Read the model definition and answer for the solid it produces. Units are mm, in the model's axes. A direction names the side the tool comes from. Round coordinates to 2 decimals unless told otherwise and drop trailing zeros. Write each loop counter-clockwise with the first axis right and the second up, starting at its lowest first coordinate (ties: lowest second). Pieces come first, ordered by that corner, then holes. Notation, with made-up numbers: (53.5, -14) - (99.5, -14) arc R7 ccw to (99.5, -2) - close; hole circle Ø4 at (80, 30). An arc over 180 degrees is marked (long way). One line per item, written item: value. Start each with the question number.
(1) The mould has two halves that part along X. Classify faces 6 (the face through (23.743, 55.535, -19.6)), 7 (the face through (-19, 53, 17)), 8 (the face through (-22.12, 55.26, -15.05)): +X half, -X half, draft (parallel to the pull), parting line (faces both ways), or undercut.
(2) A cutting plane is placed at B-B, the plane z = 0. Determine the outline of the cut face in (x, y).
(3) Find the intervals of material crossed by L1, parallel to X at y = 6.5, z = 0; L2, parallel to Y at x = -6.5, z = 21; L3, parallel to X at y = 4.25, z = -25, in increasing order.
(4) A cutting plane is placed at C-C, the plane x = -26. Determine the outline of the cut face in (y, z).
(5) For faces 1 (the face through (15.05, 55.26, -22.12)), 2 (the face through (0.66, 27.094, -14.985)), 3 (the face through (-5.865, 54.181, 14.366)), 4 (the face through (-18.684, 55.535, -19.6)), 5 (the face through (18.5, 53, 18.5)), determine the directions among +Z, -Z, +X, -X, +Y, -Y from which every point of the face is accessible in a straight line to the end or side of a thin tool.
(6) A cutting plane is placed at A-A, the plane x = 0. Determine the outline of the cut face in (y, z).
(7) A cutting plane is placed at D-D, the plane y = 51.5. Determine the outline of the cut face in (x, z).
(8) Flat-ended cylindrical pins translate along their axes: pin 1 Ø5.5 at (x, z) = (25, 0) entering from -Y; pin 2 Ø9.5 at (x, z) = (21.21, 21.21) entering from -Y; pin 3 Ø1.5 at (x, z) = (17.5, -5) entering from +Y; pin 4 Ø1 at (y, z) = (49.5, -5.5) entering from +X. Find the tip coordinate at first contact, or state that the pin passes through.
from build123d import *

# Parameters (mm, degrees)
SKETCH1_R           = 37.5
BOSS_EXTRUDE1_DEPTH = 8
SKETCH2_R           = 3
CUT_EXTRUDE1_DEPTH  = 54.633012222
SKETCH3_R           = 15
BOSS_EXTRUDE2_DEPTH = 50
BOSS_EXTRUDE4_START = -5
BOSS_EXTRUDE4_DEPTH = 5
CUT_EXTRUDE2_REACH  = 80.591
SKETCH5_R           = 3
FILLET1_R           = 5


with BuildPart() as part:
    # Sketch1 → Boss-Extrude1 (new body)
    with BuildSketch(Plane(origin=(0, 0, 0), x_dir=(1, 0, 0), z_dir=(0, 1, 0))):
        with Locations(Location((0, 0, 0), (0, 0, 270))):
            Circle(SKETCH1_R)
    extrude(amount=BOSS_EXTRUDE1_DEPTH)

    # Sketch2 → Cut-Extrude1 (cut, through all)
    with BuildSketch(Plane(origin=(0, 8, 0), x_dir=(1, 0, 0), z_dir=(0, 1, 0))):
        with Locations(Location((25, 0, 0), (0, 0, 270))):
            Circle(SKETCH2_R)
        with Locations(Location((0, 25, 0), (0, 0, 270))):
            Circle(SKETCH2_R)
        with Locations(Location((-25, 0, 0), (0, 0, 270))):
            Circle(SKETCH2_R)
        with Locations(Location((0, -25, 0), (0, 0, 270))):
            Circle(SKETCH2_R)
    extrude(amount=-CUT_EXTRUDE1_DEPTH, mode=Mode.SUBTRACT)

    # Sketch3 → Boss-Extrude2 (add)
    with BuildSketch(Plane(origin=(0, 8, 0), x_dir=(1, 0, 0), z_dir=(0, 1, 0))):
        with Locations(Location((0, 0, 0), (0, 0, 270))):
            Circle(SKETCH3_R)
    extrude(amount=BOSS_EXTRUDE2_DEPTH)

    # Sketch7 → Boss-Extrude4 (add)
    with BuildSketch(Plane(origin=(0, 58, 0), x_dir=(1, 0, 0), z_dir=(0, 1, 0)).offset(BOSS_EXTRUDE4_START)):
        with BuildLine():
            ThreePointArc((-6.464466094, -13.535533906), (-10.606601718, -10.606601718), (-13.535533906, -6.464466094))
            Line((-13.535533906, -6.464466094), (-28.284271247, -21.213203436))
            Line((-28.284271247, -21.213203436), (-21.213203436, -28.284271247))
            Line((-21.213203436, -28.284271247), (-6.464466094, -13.535533906))
        make_face()
        with BuildLine():
            Line((0, -7.071067812), (-7.071067812, 0))
            Line((-7.071067812, 0), (-13.535533906, -6.464466094))
            ThreePointArc((-13.535533906, -6.464466094), (-10.606601718, -10.606601718), (-6.464466094, -13.535533906))
            Line((-6.464466094, -13.535533906), (0, -7.071067812))
        make_face()
        with BuildLine():
            ThreePointArc((13.535533906, -6.464466094), (10.606601718, -10.606601718), (6.464466094, -13.535533906))
            Line((6.464466094, -13.535533906), (21.213203436, -28.284271247))
            Line((21.213203436, -28.284271247), (28.284271247, -21.213203436))
            Line((28.284271247, -21.213203436), (13.535533906, -6.464466094))
        make_face()
        Polygon((0, 7.071067812), (-7.071067812, 0), (0, -7.071067812), (7.071067812, 0), align=None)
        with BuildLine():
            Line((7.071067812, 0), (0, -7.071067812))
            Line((0, -7.071067812), (6.464466094, -13.535533906))
            ThreePointArc((6.464466094, -13.535533906), (10.606601718, -10.606601718), (13.535533906, -6.464466094))
            Line((13.535533906, -6.464466094), (7.071067812, 0))
        make_face()
        with BuildLine():
            Line((21.213203436, 28.284271247), (6.464466094, 13.535533906))
            ThreePointArc((6.464466094, 13.535533906), (10.606601718, 10.606601718), (13.535533906, 6.464466094))
            Line((13.535533906, 6.464466094), (28.284271247, 21.213203436))
            Line((28.284271247, 21.213203436), (21.213203436, 28.284271247))
        make_face()
        with BuildLine():
            Line((6.464466094, 13.535533906), (0, 7.071067812))
            Line((0, 7.071067812), (7.071067812, 0))
            Line((7.071067812, 0), (13.535533906, 6.464466094))
            ThreePointArc((13.535533906, 6.464466094), (10.606601718, 10.606601718), (6.464466094, 13.535533906))
        make_face()
        with BuildLine():
            Line((-21.213203436, 28.284271247), (-28.284271247, 21.213203436))
            Line((-28.284271247, 21.213203436), (-13.535533906, 6.464466094))
            ThreePointArc((-13.535533906, 6.464466094), (-10.606601718, 10.606601718), (-6.464466094, 13.535533906))
            Line((-6.464466094, 13.535533906), (-21.213203436, 28.284271247))
        make_face()
        with BuildLine():
            ThreePointArc((-6.464466094, 13.535533906), (-10.606601718, 10.606601718), (-13.535533906, 6.464466094))
            Line((-13.535533906, 6.464466094), (-7.071067812, 0))
            Line((-7.071067812, 0), (0, 7.071067812))
            Line((0, 7.071067812), (-6.464466094, 13.535533906))
        make_face()
    extrude(amount=BOSS_EXTRUDE4_DEPTH)

    # Sketch5 → Cut-Extrude2 (cut, up to next)
    with BuildSketch(Plane(origin=(0, 58, 0), x_dir=(1, 0, 0), z_dir=(0, 1, 0)), mode=Mode.PRIVATE) as cut_extrude2_sk1:
        with Locations(Location((21.213203436, -21.213203436, 0), (0, 0, 270))):
            Circle(SKETCH5_R)
    cut_extrude2_tool1 = extrude(cut_extrude2_sk1.sketch, amount=-CUT_EXTRUDE2_REACH, mode=Mode.PRIVATE) & part.part
    # Sketch5 → Cut-Extrude2 (cut, up to next)
    with BuildSketch(Plane(origin=(0, 58, 0), x_dir=(1, 0, 0), z_dir=(0, 1, 0)), mode=Mode.PRIVATE) as cut_extrude2_sk2:
        with Locations(Location((-21.213203436, 21.213203436, 0), (0, 0, 270))):
            Circle(SKETCH5_R)
    cut_extrude2_tool2 = extrude(cut_extrude2_sk2.sketch, amount=-CUT_EXTRUDE2_REACH, mode=Mode.PRIVATE) & part.part
    # Sketch5 → Cut-Extrude2 (cut, up to next)
    with BuildSketch(Plane(origin=(0, 58, 0), x_dir=(1, 0, 0), z_dir=(0, 1, 0)), mode=Mode.PRIVATE) as cut_extrude2_sk3:
        with Locations(Location((-21.213203436, -21.213203436, 0), (0, 0, 270))):
            Circle(SKETCH5_R)
    cut_extrude2_tool3 = extrude(cut_extrude2_sk3.sketch, amount=-CUT_EXTRUDE2_REACH, mode=Mode.PRIVATE) & part.part
    # Sketch5 → Cut-Extrude2 (cut, up to next)
    with BuildSketch(Plane(origin=(0, 58, 0), x_dir=(1, 0, 0), z_dir=(0, 1, 0)), mode=Mode.PRIVATE) as cut_extrude2_sk4:
        with Locations(Location((21.213203436, 21.213203436, 0), (0, 0, 270))):
            Circle(SKETCH5_R)
    cut_extrude2_tool4 = extrude(cut_extrude2_sk4.sketch, amount=-CUT_EXTRUDE2_REACH, mode=Mode.PRIVATE) & part.part
    add(cut_extrude2_tool1.solids().sort_by_distance((21.213203, 58, 21.213203))[0], mode=Mode.SUBTRACT)
    add(cut_extrude2_tool2.solids().sort_by_distance((-21.213203, 58, -21.213203))[0], mode=Mode.SUBTRACT)
    add(cut_extrude2_tool3.solids().sort_by_distance((-21.213203, 58, 21.213203))[0], mode=Mode.SUBTRACT)
    add(cut_extrude2_tool4.solids().sort_by_distance((21.213203, 58, -21.213203))[0], mode=Mode.SUBTRACT)

    # Fillet1
    fillet1_edges = [part.edges().sort_by_distance(p)[0] for p in [
        (-10.606601718, 53, 10.606601718),
        (-10.606601718, 53, -10.606601718),
        (10.606601718, 53, -10.606601718),
        (10.606601718, 53, 10.606601718),
        (13.535533906, 55.5, 6.464466094),
        (-13.535533906, 55.5, 6.464466094),
        (-6.464466094, 55.5, -13.535533906),
        (6.464466094, 55.5, -13.535533906),
        (6.464466094, 55.5, 13.535533906),
        (-6.464466094, 55.5, 13.535533906),
        (-13.535533906, 55.5, -6.464466094),
        (13.535533906, 55.5, -6.464466094),
    ]]
    fillet(fillet1_edges, radius=FILLET1_R)


solid = part.part
Here are the results:
1. face 6: undercut
1. face 7: draft
1. face 8: -X half
2. outline: (-37.5, 0) - (-28, 0) - (-28, 8) - (-37.5, 8) - close; (-22, 0) - (22, 0) - (22, 8) - (15, 8) - (15, 58) - (-15, 58) - (-15, 8) - (-22, 8) - close; (28, 0) - (37.5, 0) - (37.5, 8) - (28, 8) - close
3. L1: -37.5 to -28, -22 to 22, 28 to 37.5
3. L2: 0 to 8
3. L3: -27.95 to -3, 3 to 27.95
4. outline: (0, -27.02) - (8, -27.02) - (8, -2.83) - (0, -2.83) - close; (0, 2.83) - (8, 2.83) - (8, 27.02) - (0, 27.02) - close; (53, -23.5) - (58, -23.5) - (58, -18.93) - (53, -18.93) - close; (53, 18.93) - (58, 18.93) - (58, 23.5) - (53, 23.5) - close
5. face 1: -Z, +Y
5. face 2: none
5. face 3: +Z, +Y
5. face 4: +Y
5. face 5: +Z, +X
6. outline: (0, -37.5) - (8, -37.5) - (8, -28) - (0, -28) - close; (0, -22) - (8, -22) - (8, -15) - (58, -15) - (58, 15) - (8, 15) - (8, 22) - (0, 22) - close; (0, 28) - (8, 28) - (8, 37.5) - (0, 37.5) - close
7. outline: (-14.76, -7.22) arc R16.43 ccw to (-7.22, -14.76) arc R5 cw to (-3.88, -14.49) arc R15 ccw to (3.88, -14.49) arc R5 cw to (7.22, -14.76) arc R16.43 ccw to (14.76, -7.22) arc R5 cw to (14.49, -3.88) arc R15 ccw to (14.49, 3.88) arc R5 cw to (14.76, 7.22) arc R16.43 ccw to (7.22, 14.76) arc R5 cw to (3.88, 14.49) arc R15 ccw to (-3.88, 14.49) arc R5 cw to (-7.22, 14.76) arc R16.43 ccw to (-14.76, 7.22) arc R5 cw to (-14.49, 3.88) arc R15 ccw to (-14.49, -3.88) arc R5 cw to start
8. pin 1: through
8. pin 2: y = 0
8. pin 3: y = 8
8. pin 4: x = 14.34
